Part model, mm, in its own coordinate system. A direction names the side the tool comes from. Give positions to 0.01 mm unless a question says otherwise; leave off trailing zeros. Order: outer loops, then holes, each group sorted by start corner. A loop starts at its lowest first (then second) coordinate and runs counter-clockwise, first axis right, second up.
1. Which spindle directions (+Z, -Z, +X, -X, +Y, -Y) get a long thin tool onto all of the face, cutting with end or side? Do faces 1 (the cylindrical face through (40.25, -12.68, 58.66)), 2 (the flat face through (0, 43.8, 29)), 3 (the flat face through (-6, 68.4, 2)), 4 (the flat face through (29, 0, -34)), 5 (the flat face through (25, -25, -42)). Say none if no direction does.
2. Slice it at C-C on x = -62.5. List the corners of the cut face in (y, z).
3. Slice it at B-B on z = 6.5. Give the number of separate pieces and of enclosed holes in the cut face, and give its area (3 significant figures).
4. Drop flat-ended pins along their axis: pin 1 Ø5 at (x, z) = (0, 70) entering from +Y; pin 2 Ø17 at (x, y) = (0, -62.5) entering from -Z; pin 3 Ø6 at (y, z) = (2.5, 3.5) entering from +X; pin 4 Ø12.5 at (x, z) = (-6, 24) entering from +Y. Give the stop position or say it passes through.
5. Probe line 1 (Y direction, x = 0, z = 63); line 2 (X direction, y = 57.5, z = 15); line 3 (Z direction, x = 52, y = -38.5). List the from-to ranges inside material, lowest first.
6. Mould opens along Y. For faces 6 (the cylindrical face through (-35.525, 32.576, 47.176)), 7 (the flat face through (33.24, -34.35, 0)), 8 (the cylindrical face through (57.003, -26.739, 21.294)) say: +Y half, -Y half, draft (parallel to the pull), parting line (faces both ways), or undercut.
7. Slice it at A-A on y = -54.5. List the corners of the cut face in (x, z).
from build123d import *

# Parameters (mm, degrees)
SZKIC1_R                        = 72.5
DODANIE_WYCI_GNI_CIE1_DEPTH     = 42
SZKIC2_R                        = 48.2
DODANIE_WYCI_GNI_CIE2_DEPTH     = 33
SZKIC4_R                        = 28.6
WYTNIJ_WYCI_GNI_CIE1_DEPTH      = 156.568312969
SZKIC5_R                        = 35
WYTNIJ_WYCI_GNI_CIE2_DEPTH      = 8
SZKIC6_W                        = 12.5
SZKIC6_H                        = 6
ZAOKR_GLENIE1_R                 = 5
SZKIC7_R                        = 5.35
WYTNIJ_WYCI_GNI_CIE3_DEPTH      = 133.546218354
SZYK_KO_OWY1_COUNT              = 12
SFAZOWANIE1_SIZE                = 2
WYTNIJ_WYCI_GNI_CIE4_DEPTH      = 40
WYTNIJ_WYCI_GNI_CIE4_DEPTH_BACK = 1.6
SZKIC8_W                        = 51
SZKIC8_H                        = 59.587656766
SZKIC9_R                        = 19
WYTNIJ_WYCI_GNI_CIE5_DEPTH      = 1.6
SZKIC14_R                       = 5.35
DODANIE_WYCI_GNI_CIE4_DEPTH     = 42
SZKIC15_R                       = 12.4
WYTNIJ_WYCI_GNI_CIE6_DEPTH      = 23
WYTNIJ_WYCI_GNI_CIE7_START      = 23
SZKIC16_R                       = 19
WYTNIJ_WYCI_GNI_CIE7_DEPTH      = 23
SZKIC17_R                       = 7.5
WYTNIJ_WYCI_GNI_CIE8_DEPTH      = 23
WYTNIJ_WYCI_GNI_CIE9_REACH      = 157.568
WYTNIJ_WYCI_GNI_CIE9_END_RADIUS = 7.5
SZKIC18_R                       = 3
SFAZOWANIE2_SIZE                = 1
WYTNIJ_WYCI_GNI_CIE10_START     = 40
SZKIC19_R                       = 2
WYTNIJ_WYCI_GNI_CIE10_DEPTH     = 88.033460159


with BuildPart() as part:
    # Szkic1 → Dodanie-wyciągnięcie1 (new body)
    with BuildSketch(Plane.XY):
        with Locations(Location((0, 0, 0), (0, 0, 180))):
            Circle(SZKIC1_R)
    extrude(amount=DODANIE_WYCI_GNI_CIE1_DEPTH)

    # Szkic2 → Dodanie-wyciągnięcie2 (add)
    with BuildSketch(Plane.XY.offset(42)):
        Circle(SZKIC2_R)
    extrude(amount=DODANIE_WYCI_GNI_CIE2_DEPTH)

    # Szkic3 → Obrót1 (revolve)
    with BuildSketch(Plane(origin=(0, 0, 0), x_dir=(0, 0, -1), z_dir=(1, 0, 0)), mode=Mode.PRIVATE) as obr_t1_sk:
        Polygon((0, 47.6), (42, 41.5), (42, 28.6), (0, 28.6), align=None)
    revolve(obr_t1_sk.sketch.rotate(Axis((0, 0, 0), (0, 0, -1)), 90), axis=Axis((0, 0, 0), (0, 0, -1)))

    # Szkic4 → Wytnij-wyciągnięcie1 (cut, through all)
    with BuildSketch(Plane.XY.offset(75)):
        Circle(SZKIC4_R)
    extrude(amount=-WYTNIJ_WYCI_GNI_CIE1_DEPTH, mode=Mode.SUBTRACT)

    # Szkic5 → Wytnij-wyciągnięcie2 (cut)
    with BuildSketch(Plane(origin=(0, 0, -42), x_dir=(-1, 0, 0), z_dir=(0, 0, -1))):
        Circle(SZKIC5_R)
    extrude(amount=-WYTNIJ_WYCI_GNI_CIE2_DEPTH, mode=Mode.SUBTRACT)

    # Szkic6 → Wycięcie-obrót1 (revolve, cut)
    with BuildSketch(Plane(origin=(0, 0, 0), x_dir=(0, 0, -1), z_dir=(1, 0, 0)), mode=Mode.PRIVATE) as wyci_cie_obr_t1_sk:
        with Locations((-58.75, 45.2)):
            Rectangle(SZKIC6_W, SZKIC6_H)
    revolve(wyci_cie_obr_t1_sk.sketch.rotate(Axis((0, 0, 78.98361655), (0, 0, -1)), 90), axis=Axis((0, 0, 78.98361655), (0, 0, -1)), mode=Mode.SUBTRACT)

    # Zaokrąglenie1
    zaokr_glenie1_edges = [part.edges().sort_by_distance(p)[0] for p in [
        (-41.5, 0, -42),
    ]]
    fillet(zaokr_glenie1_edges, radius=ZAOKR_GLENIE1_R)

    # Szkic7 → Wytnij-wyciągnięcie3 (cut, through all)
    with BuildSketch(Plane.XY.offset(42)):
        with Locations((0, 62.5)):
            Circle(SZKIC7_R)
    wytnij_wyci_gni_cie3 = extrude(amount=-WYTNIJ_WYCI_GNI_CIE3_DEPTH, mode=Mode.SUBTRACT)

    # Szyk kołowy1: Wytnij-wyciągnięcie3 ×12 about axis
    szyk_ko_owy1_axis = Axis((0, 0, 0), (0, 0, 1))
    for i in range(1, SZYK_KO_OWY1_COUNT):
        add(wytnij_wyci_gni_cie3.rotate(szyk_ko_owy1_axis, i * 360 / SZYK_KO_OWY1_COUNT), mode=Mode.SUBTRACT)

    # Sfazowanie1
    sfazowanie1_edges = [part.edges().sort_by_distance(p)[0] for p in [
        (-28.6, 0, 75),
    ]]
    chamfer(sfazowanie1_edges, length=SFAZOWANIE1_SIZE)

    # Szkic8 → Wytnij-wyciągnięcie4 (cut, two sides: drawn at the far end of the back side and taken through both)
    with BuildSketch(Plane(origin=(0, 70, 0), x_dir=(1, 0, 0), z_dir=(0, 1, 0)).offset(-WYTNIJ_WYCI_GNI_CIE4_DEPTH_BACK)):
        with Locations((0, -20.8972819)):
            Rectangle(SZKIC8_W, SZKIC8_H)
    extrude(amount=WYTNIJ_WYCI_GNI_CIE4_DEPTH + WYTNIJ_WYCI_GNI_CIE4_DEPTH_BACK, mode=Mode.SUBTRACT)

    # Szkic9 → Wytnij-wyciągnięcie5 (cut)
    with BuildSketch(Plane(origin=(0, 68.4, 0), x_dir=(1, 0, 0), z_dir=(0, 1, 0))):
        with Locations(Location((0.027670653, -21, 0), (0, 0, 270))):
            Circle(SZKIC9_R)
    extrude(amount=-WYTNIJ_WYCI_GNI_CIE5_DEPTH, mode=Mode.SUBTRACT)

    # Szkic14 → Dodanie-wyciągnięcie4 (add)
    with BuildSketch(Plane.XY.offset(42)):
        with Locations((0, 62.5)):
            Circle(SZKIC14_R)
    extrude(amount=-DODANIE_WYCI_GNI_CIE4_DEPTH)

    # Szkic15 → Wytnij-wyciągnięcie6 (cut)
    with BuildSketch(Plane(origin=(0, 66.8, 0), x_dir=(1, 0, 0), z_dir=(0, 1, 0))):
        with Locations(Location((0.027670653, -21, 0), (0, 0, 270))):
            Circle(SZKIC15_R)
    extrude(amount=-WYTNIJ_WYCI_GNI_CIE6_DEPTH, mode=Mode.SUBTRACT)

    # Szkic16 → Wytnij-wyciągnięcie7 (cut)
    with BuildSketch(Plane(origin=(0, 66.8, 0), x_dir=(1, 0, 0), z_dir=(0, 1, 0)).offset(WYTNIJ_WYCI_GNI_CIE7_START)):
        with Locations(Location((0.027670653, -21, 0), (0, 0, 270))):
            Circle(SZKIC16_R)
    extrude(amount=-WYTNIJ_WYCI_GNI_CIE7_DEPTH, mode=Mode.SUBTRACT)

    # Szkic17 → Wytnij-wyciągnięcie8 (cut)
    with BuildSketch(Plane(origin=(0, 43.8, 0), x_dir=(1, 0, 0), z_dir=(0, 1, 0))):
        with Locations(Location((0.027670653, -21, 0), (0, 0, 270))):
            Circle(SZKIC17_R)
    extrude(amount=-WYTNIJ_WYCI_GNI_CIE8_DEPTH, mode=Mode.SUBTRACT)

    # Wytnij-wyciągnięcie9: up to this cylinder (the profile starts outside it)
    wytnij_wyci_gni_cie9_end = Plane(origin=(0.027670653, 39, 21), z_dir=(0, 1, 0)) * Cylinder(WYTNIJ_WYCI_GNI_CIE9_END_RADIUS, 331.136, mode=Mode.PRIVATE)
    # Szkic18 → Wytnij-wyciągnięcie9 (cut, up to the surface)
    with BuildSketch(Plane.XY.offset(75), mode=Mode.PRIVATE) as wytnij_wyci_gni_cie9_sk1:
        with Locations((0, 39)):
            Circle(SZKIC18_R)
    wytnij_wyci_gni_cie9_tool1 = extrude(wytnij_wyci_gni_cie9_sk1.sketch, amount=-WYTNIJ_WYCI_GNI_CIE9_REACH, mode=Mode.PRIVATE) - wytnij_wyci_gni_cie9_end
    add(wytnij_wyci_gni_cie9_tool1.solids().sort_by_distance((0, 39, 75))[0], mode=Mode.SUBTRACT)

    # Sfazowanie2
    sfazowanie2_edges = [part.edges().sort_by_distance(p)[0] for p in [
        (-3, 39, 75),
    ]]
    chamfer(sfazowanie2_edges, length=SFAZOWANIE2_SIZE)

    # Szkic19 → Wytnij-wyciągnięcie10 (cut, through all)
    with BuildSketch(Plane(origin=(0, 0, 0), x_dir=(1, 0, 0), z_dir=(0, 1, 0)).offset(WYTNIJ_WYCI_GNI_CIE10_START)):
        with Locations(Location((0, -70, 0), (0, 0, 90))):
            Circle(SZKIC19_R)
    extrude(amount=WYTNIJ_WYCI_GNI_CIE10_DEPTH, mode=Mode.SUBTRACT)


solid = part.part
Data:
1. face 1: none
1. face 2: +Y
1. face 3: +Z, -Z, +X, -X, +Y
1. face 4: -Z
1. face 5: -Z, +X, -X, +Y, -Y
2. outline: (-36.74, 0) - (-5.35, 0) - (-5.35, 42) - (-36.74, 42) - close; (5.35, 0) - (36.74, 0) - (36.74, 42) - (5.35, 42) - close
3. separate pieces: 1
3. enclosed holes: 12
3. area: 12,800 mm2
4. pin 1: stops at y = 48.2
4. pin 2: stops at z = 0
4. pin 3: stops at x = 72.5
4. pin 4: stops at y = 66.8
5. line 1: y = -42.2 to -28.6, 28.6 to 36, 42 to 42.2
5. line 2: x = -44.16 to -35.4, -27.1 to -10.82, 10.88 to 27.1, 35.4 to 44.16
5. line 3: z = 0 to 42
6. face 6: parting line
6. face 7: draft
6. face 8: undercut
7. outline: (-47.81, 0) - (-36.59, 0) - (-36.59, 42) - (-47.81, 42) - close; (-25.91, 0) - (25.91, 0) - (25.91, 42) - (-25.91, 42) - close; (36.59, 0) - (47.81, 0) - (47.81, 42) - (36.59, 42) - close
